Check sheet for the modelled part. Datum: model origin and axes. Units: mm. A direction names the side the tool comes from. Round coordinates to 2 decimals unless told otherwise and drop trailing zeros. Order: outer loops, then holes, each group sorted by start corner. A loop starts at its lowest first (then second) coordinate and runs counter-clockwise, first axis right, second up.
(1) Mould release check, pull along Y, two halves, no side actions. Record for faces 6 (the cylindrical face through (1.4, 0.06, -17.02)), 7 (the cylindrical face through (-2.17, 9.76, 2.99)), 8 (the flat face through (-1, -5, 0)): released by +Y, released by -Y, zero draft, split by the parting line, or undercut.
(2) Sectioned sample at A-A, the plane x = 0. Enter the section's corners in (y, z).
(3) Sectioned sample at C-C, the plane x = 6. Enter the section's corners in (y, z).
(4) Tool access check on faces 1 (the cylindrical face through (-2.562, 5.974, 0.986)), 2 (the flat face through (1.1, 1.1, -18.5)), 3 (the cylindrical face through (2.697, -5.914, 0.986)), 4 (the cylindrical face through (-0.878, 3.954, -5.886)), 5 (the flat face through (4.3, 0.1, 4)). Record the directions out of +Z, -Z, +X, -X, +Y, -Y that give a thin tool (end or side, any length) a straight path to the whole face; none if there is none.
(5) Depth check by flat-ended pin: pin 1 (5 mm diameter, centred on y = -3.5, z = -5.5, fed in from +X); pin 2 (10 mm diameter, centred on x = -6.5, z = 1, fed in from +Y); pin 3 (1 mm diameter, centred on x = 5.5, z = -15, fed in from -Y); pin 4 (8 mm diameter, centred on y = 3.5, z = -14, fed in from +X). Enter the tip coordinate at first touch or a pass-through.
(6) Sectioned sample at D-D, the plane z = -8.5. Enter the section's corners in (x, y), and give its area (3 significant figures).
(7) Thickness scan on probe 1 along Z at (x, y) = (-2, -2.5); probe 2 along Y at (x, z) = (0, -1); probe 3 along Z at (x, y) = (-0.75, 5.5). Record the ranges inside material, lowest first.
Autodesk Inventor part; units mm, degrees
ref_plane "Arbeitsebene2" through (-24.4207, -24.3793, -13.5) normal (0, 0, -1) x (0, 1, 0)
ref_plane "Arbeitsebene3" through (-24.4207, -24.3793, -18.5) normal (0, 0, -1) x (0, 1, 0)
ref_plane "YZ Plane" through (0, 0, 0) normal (1, 0, 0) x (0, 1, 0)
ref_plane "Arbeitsebene2" through (-24.4207, -24.3793, -13.5) normal (0, 0, -1) x (0, 1, 0)
ref_plane "Arbeitsebene3" through (-24.4207, -24.3793, -18.5) normal (0, 0, -1) x (0, 1, 0)
sketch "Skizze1" plane through (0, 0, 0) normal (0, 0, 1) x (1, 0, 0)
  arc A0 (-2.8009, 5.3061) -> (2.8009, 5.3061) centre (0, 0) ccw
  circle A1 centre (0, 0) radius 5
  circle A2 centre (0, 0) radius 4.8
  circle A3 centre (0, 0) radius 4.05
  circle A4 centre (0, 0) radius 10
  point P0 (0, 0)
  dimension "d0" = 0.2
  dimension "d1" = 8.1
  dimension "d14" = 20
extrude "Extrusion1" add sketch "Skizze1" against normal up to surface (18.5 mm away) contours A2
sketch "Skizze2" plane through (0, 0, 0) normal (0, 0, 1) x (1, 0, 0)
  circle A0 centre (0, 0) radius 4.8
  circle A1 centre (0, 0) radius 4.05
  arc A2 (2.3233, 6.0706) -> (-5.9453, 2.6275) centre (0, 0) ccw
  circle A3 centre (0, 0) radius 6.5
  point P0 (-5.9453, 2.6275)
  point P1 (2.3233, 6.0706)
extrude "Extrusion2" add sketch "Skizze2" along normal blind 2 contours A0 | A3 A2
sketch "Skizze4" plane through (0, 0, -18.5) normal (0, 0, -1) x (-1, 0, 0)
  circle A0 centre (0, 0) radius 4.05
  circle A1 centre (0, 0) radius 1.4
  point P0 (0, 0)
  dimension "d16" = 2.8
extrude "Extrusion4" add sketch "Skizze4" against normal blind 3
sketch "Skizze5" plane through (0, 0, 2) normal (0, 0, 1) x (1, 0, 0)
  circle A0 centre (0, 0) radius 6.5
  circle A1 centre (0, 0) radius 6.5
  circle A2 centre (0, 0) radius 4.05
  circle A3 centre (0, 0) radius 10
  point P0 (0, 0)
  dimension "d19" = 20
extrude "Extrusion5" add sketch "Skizze5" along normal blind 2 contours A0 | A3
properties part number "50_ETL_Motionpart1_v0"
Derived:
1. face 6: undercut
1. face 7: split by the parting line
1. face 8: zero draft
2. outline: (-10, 2) - (-6.5, 2) - (-6.5, 0) - (-4.8, 0) - (-4.8, -18.5) - (-1.4, -18.5) - (-1.4, -15.5) - (-4.05, -15.5) - (-4.05, 4) - (-10, 4) - close; (1.4, -18.5) - (4.8, -18.5) - (4.8, 0) - (6.5, 0) - (6.5, 2) - (10, 2) - (10, 4) - (4.05, 4) - (4.05, -15.5) - (1.4, -15.5) - close
3. outline: (-8, 2) - (-2.5, 2) - (-2.5, 0) - (2.5, 0) - (2.5, 2) - (8, 2) - (8, 4) - (-8, 4) - close
4. face 1: -Z, +Y
4. face 2: -Z, +X, -X, +Y, -Y
4. face 3: -Z
4. face 4: +Z
4. face 5: +Z, +X, -X, +Y, -Y
5. pin 1: stops at x = 4.69
5. pin 2: stops at y = 9.87
5. pin 3: passes through
5. pin 4: stops at x = 4.8
6. outline: circle Ø9.6 at (0, 0); hole circle Ø8.1 at (0, 0)
6. area: 20.9 mm2
7. probe 1: z = -18.5 to -15.5
7. probe 2: y = -4.8 to -4.05, 4.05 to 4.8
7. probe 3: z = 0 to 4
